Geometry: see drawing. Coordinates: mm, zero at the bounding-box minimum. A direction names the side the tool comes from. Round coordinates to 2 decimals unless told otherwise and drop trailing zeros. Loops run counter-clockwise (first coordinate to the right, second up) from the corner with the lowest first, then second, coordinate; pieces in that order, holes last. Notation, with made-up numbers: (54, -13) -> (94, -13) arc R15 ccw to (94, 15) -> close; hole circle Ø9 at (55.25, 67). An arc over 180 degrees is marked (long way). Answer in a Markdown table with one row per item.
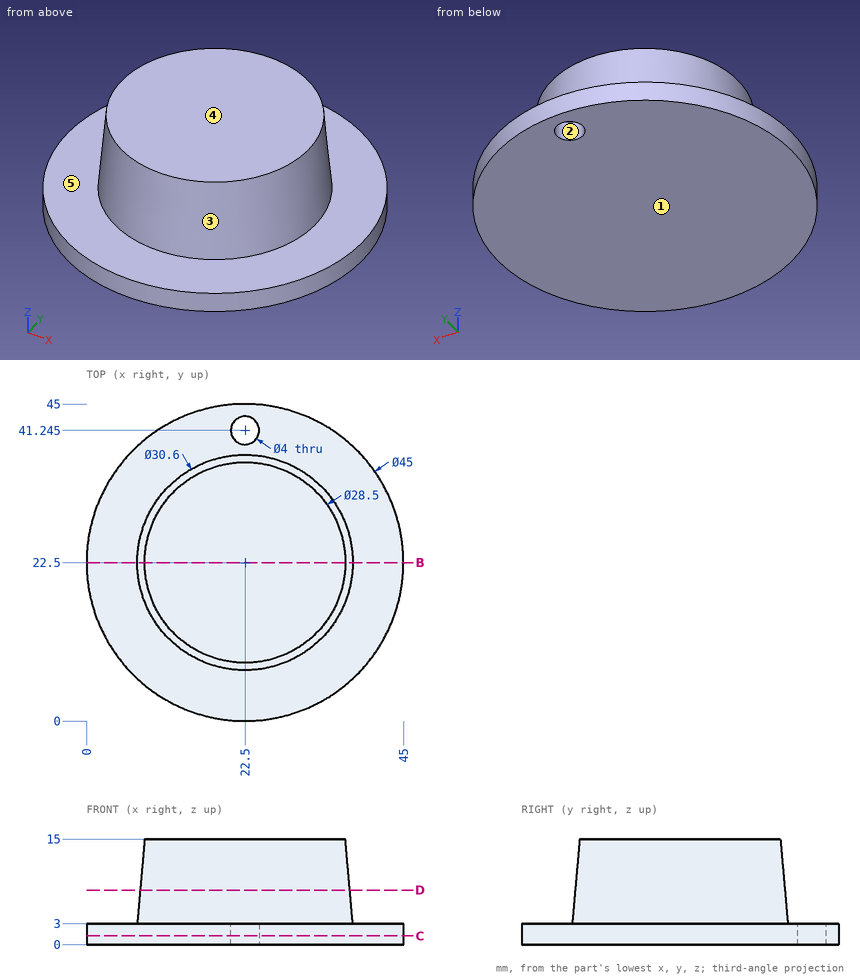
Item 1: Section query C-C, the plane z = 1.25. Output: boundary loops of the cut face in (x, y) (1 decimal), and give its area (3 significant figures).
Ans:
| item | result |
|---|---|
| outline | circle Ø45 at (22.5, 22.5); hole circle Ø4 at (22.5, 41.2) |
| area | 1,580 mm2 |
Item 2: Set-up query: the marked faces 4 and 5. Return all of +Z, -Z, +X, -X, +Y, -Y with unobstructed straight access to the full face (end or side cutting, diameter ignored); none if empty.
Ans:
| item | result |
|---|---|
| face 4 | +Z, +X, -X, +Y, -Y |
| face 5 | +Z |
Item 3: First-contact query: P1, Ø1, axis at x = 18, z = 13.5, coming from the +Y side; P2, Ø4, axis at x = 40.5, y = 5, coming from the +Z side; P3, Ø6, axis at x = 25, z = 3.5, coming from the +Y side; P4, Ø5, axis at x = 22, z = 5, coming from the -Y side. Flat tips, straight axial feed; report the tip coordinate or a pass-through.
Ans:
| item | result |
|---|---|
| P1 | y = 36.32 |
| P2 | through |
| P3 | y = 45 |
| P4 | y = 0 |
Item 4: Ray query, L1, parallel to Y at x = 22.5, z = 1.05 (1 decimal); L2, parallel to Z at x = 16.5, y = 43.5; L3, parallel to X at y = 20, z = 6. Return the intervals inside material, ascending.
Ans:
| item | result |
|---|---|
| L1 | 0 to 39.2, 43.2 to 45 |
| L2 | 0 to 3 |
| L3 | 7.67 to 37.33 |
Item 5: Section query D-D, the plane z = 7.75. Output: boundary loops of the cut face in (x, y) (1 decimal).
Ans:
| item | result |
|---|---|
| outline | circle Ø29.8 at (22.5, 22.5) |
Item 6: Section query B-B, the plane y = 22.5. Output: boundary loops of the cut face in (x, z), and give its area (3 significant figures).
Ans:
| item | result |
|---|---|
| outline | (0, 0) -> (45, 0) -> (45, 3) -> (37.8, 3) -> (36.75, 15) -> (8.25, 15) -> (7.2, 3) -> (0, 3) -> close |
| area | 490 mm2 |
Item 7: Mould query, pull axis Y, two halves, no side actions, for the marked faces 1, 2 and 3. Classes: released by +Y, released by -Y, zero draft, split by the parting line, or undercut.
Ans:
| item | result |
|---|---|
| face 1 | zero draft |
| face 2 | undercut |
| face 3 | split by the parting line |
